Autodesk Inventor part; units mm, degrees
ref_plane "to_frame_XY" through (0, 0, 0) normal (0, 0, 1) x (1, 0, 0)
ref_plane "to_frame_YZ" through (0, 0, 0) normal (1, 0, 0) x (0, 1, 0)
ref_plane "to_frame_ZX" through (0, 0, 0) normal (0, 1, 0) x (0, 0, 1)
sketch "Sketch_5" plane through (0, 0, 0) normal (0, 0, 1) x (1, 0, 0)
  arc A0 (-10, 3.3) -> (-9.7, 3) centre (-9.7, 3.3) ccw
  line L0 (-9.7, 3) -> (-8, 3)
  line L1 (-8, 3) -> (-8, 6)
  line L2 (-8, 6) -> (-7.0607, 6)
  line L3 (-7.0607, 6) -> (-4, 2.9393)
  line L4 (-4, 2.9393) -> (-4, 0.3)
  line L5 (-4, 0.3) -> (-3.7, 0)
  line L6 (-3.7, 0) -> (-4, -0.3)
  line L7 (-4, -0.3) -> (-4, -2.9393)
  line L8 (-4, -2.9393) -> (-7.0607, -6)
  line L9 (-7.0607, -6) -> (-8, -6)
  line L10 (-8, -6) -> (-8, -3)
  line L11 (-8, -3) -> (-9.7, -3)
  arc A1 (-9.7, -3) -> (-10, -3.3) centre (-9.7, -3.3) ccw
  line L12 (-10, -3.3) -> (-10, -9)
  arc A2 (-10, -9) -> (-9, -10) centre (-9, -9) ccw
  line L13 (-9, -10) -> (-3.3, -10)
  arc A3 (-3.3, -10) -> (-3, -9.7) centre (-3.3, -9.7) ccw
  line L14 (-3, -9.7) -> (-3, -8)
  line L15 (-3, -8) -> (-6, -8)
  line L16 (-6, -8) -> (-6, -7.0607)
  line L17 (-6, -7.0607) -> (-2.9393, -4)
  line L18 (-2.9393, -4) -> (-0.3, -4)
  line L19 (-0.3, -4) -> (0, -3.7)
  line L20 (0, -3.7) -> (0.3, -4)
  line L21 (0.3, -4) -> (2.9393, -4)
  line L22 (2.9393, -4) -> (6, -7.0607)
  line L23 (6, -7.0607) -> (6, -8)
  line L24 (6, -8) -> (3, -8)
  line L25 (3, -8) -> (3, -9.7)
  arc A4 (3, -9.7) -> (3.3, -10) centre (3.3, -9.7) ccw
  line L26 (3.3, -10) -> (9, -10)
  arc A5 (9, -10) -> (10, -9) centre (9, -9) ccw
  line L27 (10, -9) -> (10, -3.3)
  arc A6 (10, -3.3) -> (9.7, -3) centre (9.7, -3.3) ccw
  line L28 (9.7, -3) -> (8, -3)
  line L29 (8, -3) -> (8, -6)
  line L30 (8, -6) -> (7.0607, -6)
  line L31 (7.0607, -6) -> (4, -2.9393)
  line L32 (4, -2.9393) -> (4, -0.3)
  line L33 (4, -0.3) -> (3.7, 0)
  line L34 (3.7, 0) -> (4, 0.3)
  line L35 (4, 0.3) -> (4, 2.9393)
  line L36 (4, 2.9393) -> (7.0607, 6)
  line L37 (7.0607, 6) -> (8, 6)
  line L38 (8, 6) -> (8, 3)
  line L39 (8, 3) -> (9.7, 3)
  arc A7 (9.7, 3) -> (10, 3.3) centre (9.7, 3.3) ccw
  line L40 (10, 3.3) -> (10, 9)
  arc A8 (10, 9) -> (9, 10) centre (9, 9) ccw
  line L41 (9, 10) -> (3.3, 10)
  arc A9 (3.3, 10) -> (3, 9.7) centre (3.3, 9.7) ccw
  line L42 (3, 9.7) -> (3, 8)
  line L43 (3, 8) -> (6, 8)
  line L44 (6, 8) -> (6, 7.0607)
  line L45 (6, 7.0607) -> (2.9393, 4)
  line L46 (2.9393, 4) -> (0.3, 4)
  line L47 (0.3, 4) -> (0, 3.7)
  line L48 (0, 3.7) -> (-0.3, 4)
  line L49 (-0.3, 4) -> (-2.9393, 4)
  line L50 (-2.9393, 4) -> (-6, 7.0607)
  line L51 (-6, 7.0607) -> (-6, 8)
  line L52 (-6, 8) -> (-3, 8)
  line L53 (-3, 8) -> (-3, 9.7)
  arc A10 (-3, 9.7) -> (-3.3, 10) centre (-3.3, 9.7) ccw
  line L54 (-3.3, 10) -> (-9, 10)
  arc A11 (-9, 10) -> (-10, 9) centre (-9, 9) ccw
  line L55 (-10, 9) -> (-10, 3.3)
  circle A12 centre (0, 0) radius 2.1
extrude "Extrusion1" add sketch "Sketch_5" against normal blind 110
ref_plane "to_frame_XY" through (0, 0, 0) normal (0, 0, 1) x (1, 0, 0)
ref_plane "to_frame_YZ" through (0, 0, 0) normal (1, 0, 0) x (0, 1, 0)
ref_plane "to_frame_ZX" through (0, 0, 0) normal (0, 1, 0) x (0, 0, 1)
properties part number "프로파일_110" material "알루미늄 6061"
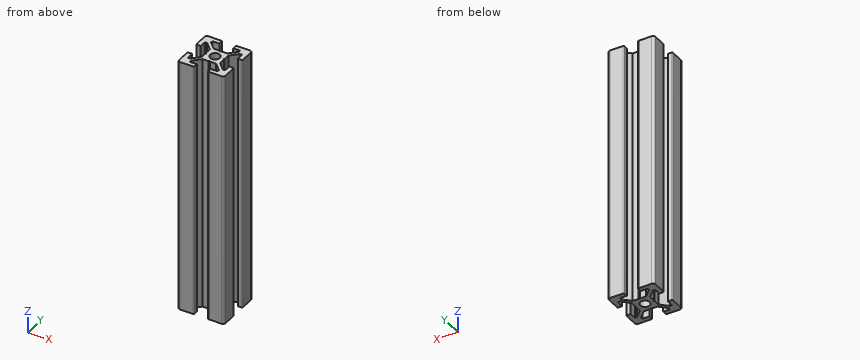
Source: CAD feature listing. Evaluate the final solid. Frame: model axes, mm. Coordinates: 2 decimals unless noted, no trailing zeros. Loops run counter-clockwise (first coordinate to the right, second up) from the corner with the lowest first, then second, coordinate; pieces in that order, holes last. Notation, with made-up numbers: M 24.5,46 L 79.5,46 A31 ccw 79.5,82 Z; hole C 76.25,9 d3. An arc over 180 degrees is marked long. Use CSV: the item, a comma, the result in double quotes.
(1) Line query: line 1 (Y direction, x = 0, z = -55.5); line 2 (X direction, y = 7.75, z = -39); line 3 (X direction, y = 4.25, z = -28.5). Output: solid intervals per line, ascending. Write a range as [from, to].
Answers follow:
line 1,"[-3.7, -2.1], [2.1, 3.7]"
line 2,"[-10, -6], [6, 10]"
line 3,"[-10, -8], [-5.31, -3.19], [3.19, 5.31], [8, 10]"
(2) Cut plane A-A on y = 5. Return loops of the section in (x, z).
Answers follow:
outline,"M -10,-110 L -8,-110 L -8,0 L -10,0 Z; M -6.06,-110 L -3.94,-110 L -3.94,0 L -6.06,0 Z; M 3.94,-110 L 6.06,-110 L 6.06,0 L 3.94,0 Z; M 8,-110 L 10,-110 L 10,0 L 8,0 Z"
(3) Contact query for flat-ended pins moving along their axis: pin 1 (1.3 mm diameter, centred on y = -1.5, z = -60.5, fed in from +X); pin 2 (0.8 mm diameter, centred on x = -1.5, z = -76, fed in from +Y); pin 3 (1.3 mm diameter, centred on x = 1.5, z = -80.5, fed in from -Y). Output: stop coordinate, or through.
Answers follow:
pin 1,"x = 4"
pin 2,"y = 4"
pin 3,"y = -4"
